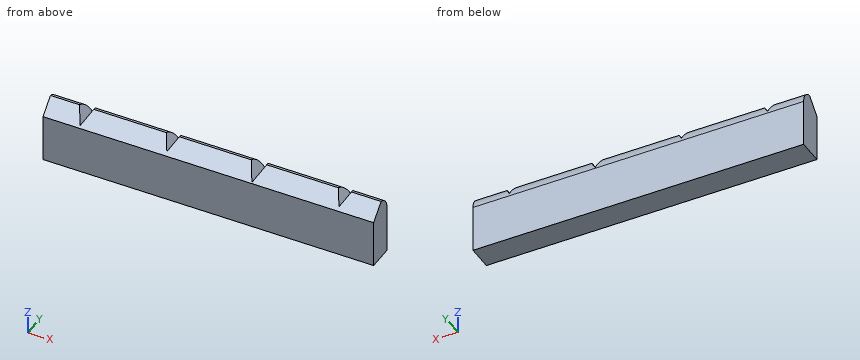
from build123d import *

# Parameters (mm, degrees)
F0_W        = 40.64
F0_H        = 3.0988
F1_DEPTH    = 7.62
F3_R        = 1.778
F4_T1_DEPTH = 49.7849047052
F5_DEPTH    = 25.4


# Not quite as in the source:
# - a fillet or chamfer that OpenCascade refuses, or shapes differently, is made with other operations: its cross-section is extruded or revolved along the edge and cut away or added


with BuildPart() as f1:
    # F0 (on Top) → F1 (new body)
    with BuildSketch(Plane.XY):
        with Locations((0, 1.5494)):
            Rectangle(F0_W, F0_H)
    extrude(amount=F1_DEPTH)

    # F3
    f3_edges = [f1.edges().sort_by_distance(p)[0] for p in [
        (0, 3.0988, 7.62),
    ]]
    fillet(f3_edges, radius=F3_R)

    # F4: chamfer of 1.778 on 1 edges, made by hand

    # F4_s2 → F4_t1 (cut)
    with BuildSketch(Plane.YZ.offset(-24.8924523526)):
        Polygon((1.778, 7.62), (0, 5.842), (0, 7.62), align=None)
    extrude(amount=F4_T1_DEPTH, mode=Mode.SUBTRACT)

    # F2 (on face) → F5 (cut)
    with BuildSketch(Plane.XZ):
        Polygon((-15.875, 6.0552954744), (-14.9716174209, 7.62), (-16.7783825791, 7.62), align=None)
        Polygon((-4.4531409051, 7.62), (-6.1132590949, 7.62), (-5.2832, 6.1822954744), align=None)
        Polygon((6.2853060633, 7.62), (4.3318939367, 7.62), (5.3086, 5.9282954744), align=None)
        Polygon((16.7050590949, 7.62), (15.0449409051, 7.62), (15.875, 6.1822954744), align=None)
    extrude(amount=-F5_DEPTH, mode=Mode.SUBTRACT)


solid = f1.part
The listing builds one solid part. Answer for the finished solid, in the listing's coordinates (mm). Give positions to 0.01 mm unless a question says otherwise; leave off trailing zeros. Loops run counter-clockwise (first coordinate to the right, second up) from the corner with the lowest first, then second, coordinate; pieces in that order, holes last. Notation, with made-up numbers: (9.25, 52) - (53.25, 52) arc R26 ccw to (53.25, 69) - close; hole circle Ø9 at (28.25, 21). An arc over 180 degrees is marked (long way). Use one line per item in the form item = value.
1. Find the intervals of material crossed by line 1 along X through (y, z) = (1.25, 6.75); line 2 along Z through (x, y) = (17, 0.5); line 3 along Y through (x, z) = (2, 6.5), in increasing order. Write a range as [from, to].
Calculated:
line_1 = [-20.32, -16.28], [-15.47, -5.61], [-4.96, 4.83], [5.78, 15.55], [16.2, 20.32]
line_2 = [0, 6.34]
line_3 = [0.66, 2.97]
2. Section B-B on x = 4 is taken. Give the vertices of the cut face in (y, z), then the cut area to 3 significant figures.
Calculated:
outline = (0, 0) - (3.1, 0) - (3.1, 5.84) arc R1.78 ccw to (1.73, 7.57) - (0, 5.84) - close
area = 21.4 mm^2
3. Section A-A on y = 0.75 is taken. Give the vertices of the cut face in (x, z) (3 decimals).
Calculated:
outline = (-20.32, 0) - (20.32, 0) - (20.32, 6.592) - (16.112, 6.592) - (15.875, 6.182) - (15.638, 6.592) - (5.692, 6.592) - (5.309, 5.928) - (4.925, 6.592) - (-5.047, 6.592) - (-5.283, 6.182) - (-5.52, 6.592) - (-15.565, 6.592) - (-15.875, 6.055) - (-16.185, 6.592) - (-20.32, 6.592) - close
